Could you check a few things on this drawing? It's one solid part, dimensions in mm from its lowest x, y, z. Give positions to 0.01 mm unless a question says otherwise; leave off trailing zeros. Order: outer loops, then holes, each group sorted by start corner. A loop starts at its lowest first (then second) coordinate and runs counter-clockwise, first axis right, second up.
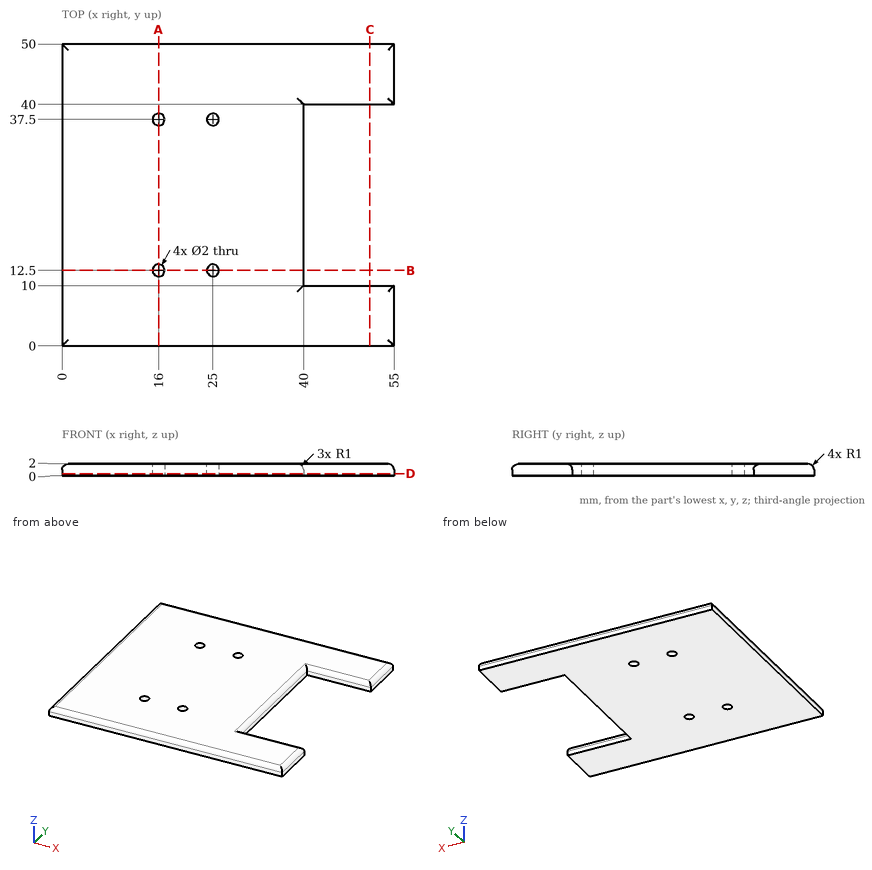
Q1. If we section it at D-D on z = 0.4: List the corners of the cut face in (x, y) for me.
Filled sheet:
outline: (0, 0) - (55, 0) - (55, 10) - (40, 10) - (40, 40) - (55, 40) - (55, 50) - (0, 50) - close; hole circle Ø2 at (16, 12.5); hole circle Ø2 at (16, 37.5); hole circle Ø2 at (25, 12.5); hole circle Ø2 at (25, 37.5)
Q2. I'm going to push flat-ended pins straight in: P1, Ø1, axis at x = 30, z = 1.5, coming from the +Y side; P2, Ø0.5, axis at y = 30, z = 0.5, coming from the +X side. Where does each tip first touch, or does it pass through?
Filled sheet:
P1: stops at y = 50
P2: stops at x = 40
Q3. If we section it at C-C on x = 51: List the corners of the cut face in (y, z) for me.
Filled sheet:
outline: (0, 0) - (10, 0) - (10, 1) arc R1 ccw to (9, 2) - (1, 2) arc R1 ccw to (0, 1) - close; (40, 0) - (50, 0) - (50, 1) arc R1 ccw to (49, 2) - (41, 2) arc R1 ccw to (40, 1) - close
Q4. I need wall thicknesses on L1, parallel to Y at x = 16, z = 0.65; L2, parallel to X at y = 37.5, z = 0.95; L3, parallel to Y at x = 46.5, z = 1.05. Which ranges of each line are inside material? Lowest first, please.
Filled sheet:
L1: y = 0 to 11.5, 13.5 to 36.5, 38.5 to 50
L2: x = 0 to 15, 17 to 24, 26 to 40
L3: y = 0 to 10, 40 to 50
Q5. If we section it at B-B on y = 12.5: List the corners of the cut face in (x, z) for me, plus the area to 3 significant figures.
Filled sheet:
outline: (0, 0) - (15, 0) - (15, 2) - (1, 2) arc R1 ccw to (0, 1) - close; (17, 0) - (24, 0) - (24, 2) - (17, 2) - close; (26, 0) - (40, 0) - (40, 1) arc R1 ccw to (39, 2) - (26, 2) - close
area: 71.6 mm2
Q6. If we section it at A-A on x = 16: List the corners of the cut face in (y, z) for me.
Filled sheet:
outline: (0, 0) - (11.5, 0) - (11.5, 2) - (1, 2) arc R1 ccw to (0, 1) - close; (13.5, 0) - (36.5, 0) - (36.5, 2) - (13.5, 2) - close; (38.5, 0) - (50, 0) - (50, 1) arc R1 ccw to (49, 2) - (38.5, 2) - close
